Could you check a few things on this model? Use its own coordinates, in mm. Face numbers are marked on the shaded views. A direction names the side the tool comes from. Coordinates: 2 decimals unless noted, no trailing zeros. Write each loop counter-clockwise with the first axis right and the second up, starting at its lowest first coordinate (ties: lowest second). Pieces come first, ordered by that corner, then holes.
Item 1: For P1, Ø6, axis at y = 7.5, z = -1, coming from the +X side; P2, Ø3.5, axis at y = 10.5, z = 2.5, coming from the -X side; P3, Ø2.5, axis at x = 13, z = -1.5, coming from the +Y side, each with a flat end and sliding along its axis, tell me the tip position at first contact or that it passes through.
Item 2: Which directions (+Z, -Z, +X, -X, +Y, -Y) give clear straight access to the entire face, cutting with the end or side of a thin tool? Please do the marked faces 1, 2, 3 and 4.
Item 3: I want a section at C-C on z = 3.5. Please give me the cut outline in (x, y), then the cut area to 3 significant figures.
Item 4: I want a section at D-D on y = 20.5. Please give me the cut outline in (x, z).
Item 5: I want a section at B-B on x = 1. Please give me the cut outline in (y, z), then the cut area to 3 significant figures.
Item 6: If I drill on probe 1 along Y at (x, z) = (8, -1.25); probe 2 along X at (y, z) = (16.4, 0); probe 3 along X at (y, z) = (13.75, 0.5), over which ranges is the centre line in solid material (lowest first)?
Item 7: I want a section at A-A on x = -14. Please give me the cut outline in (y, z).
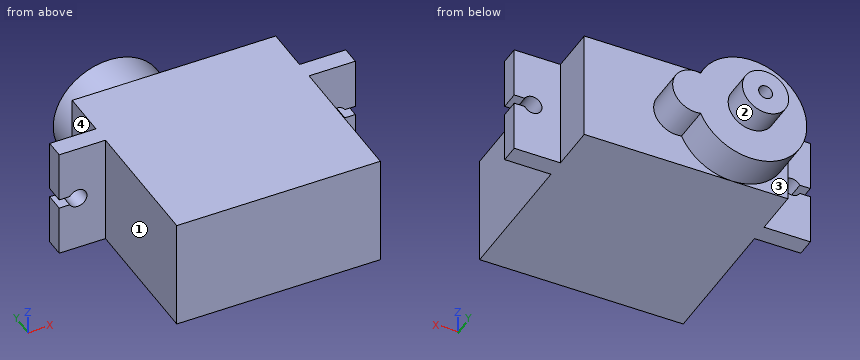
from build123d import *

# Parameters (mm, degrees)
SKETCH1_W           = 22
SKETCH1_H           = 12
BOSS_EXTRUDE1_DEPTH = 22
BOSS_EXTRUDE2_DEPTH = 4
SKETCH3_W           = 5
SKETCH3_H           = 2
BOSS_EXTRUDE3_DEPTH = 12
CUT_EXTRUDE1_REACH  = 26.104
SKETCH5_R           = 2.5
SKETCH5_R_2         = 0.75
BOSS_EXTRUDE4_DEPTH = 3


with BuildPart() as part:
    # Sketch1 → Boss-Extrude1 (new body)
    with BuildSketch(Plane(origin=(0, 0, 0), x_dir=(1, 0, 0), z_dir=(0, 1, 0))):
        Rectangle(SKETCH1_W, SKETCH1_H)
    extrude(amount=BOSS_EXTRUDE1_DEPTH)

    # Sketch2 → Boss-Extrude2 (add)
    with BuildSketch(Plane(origin=(0, 22, 0), x_dir=(1, 0, 0), z_dir=(0, 1, 0))):
        with BuildLine():
            ThreePointArc((0.479166667, 2.445144707), (-11, 0), (0.479166667, -2.445144707))
            ThreePointArc((0.479166667, -2.445144707), (3.5, 0), (0.479166667, 2.445144707))
        make_face()
    extrude(amount=BOSS_EXTRUDE2_DEPTH)

    # Sketch3 → Boss-Extrude3 (add)
    with BuildSketch(Plane.XY.offset(6)):
        with Locations((13.5, 16)):
            Rectangle(SKETCH3_W, SKETCH3_H)
    boss_extrude3 = extrude(amount=-BOSS_EXTRUDE3_DEPTH)

    # Sketch4 → Cut-Extrude1 (cut, up to next)
    with BuildSketch(Plane(origin=(0, 17, 0), x_dir=(1, 0, 0), z_dir=(0, 1, 0)), mode=Mode.PRIVATE) as cut_extrude1_sk1:
        with BuildLine():
            Line((14.866025404, 0.5), (16, 0.5))
            Line((16, 0.5), (16, -0.5))
            Line((16, -0.5), (14.866025404, -0.5))
            ThreePointArc((14.866025404, -0.5), (13, 0), (14.866025404, 0.5))
        make_face()
    cut_extrude1_tool1 = extrude(cut_extrude1_sk1.sketch, amount=-CUT_EXTRUDE1_REACH, mode=Mode.PRIVATE) & part.part
    cut_extrude1 = cut_extrude1_tool1.solids().sort_by_distance((14.368381, 17, 0))[0]
    add(cut_extrude1, mode=Mode.SUBTRACT)

    # Mirror1: Boss-Extrude3, Cut-Extrude1 across plane
    add(boss_extrude3.mirror(Plane(origin=(0, 0, 0), x_dir=(0, 0, 1), z_dir=(1, 0, 0))))
    add(cut_extrude1.mirror(Plane(origin=(0, 0, 0), x_dir=(0, 0, 1), z_dir=(1, 0, 0))), mode=Mode.SUBTRACT)

    # Sketch5 → Boss-Extrude4 (add)
    with BuildSketch(Plane(origin=(0, 26, 0), x_dir=(1, 0, 0), z_dir=(0, 1, 0))):
        with Locations(Location((-5, 0, 0), (0, 0, 270))):
            Circle(SKETCH5_R)
        with Locations(Location((-5, 0, 0), (0, 0, 270))):
            Circle(SKETCH5_R_2, mode=Mode.SUBTRACT)
    extrude(amount=BOSS_EXTRUDE4_DEPTH)


solid = part.part
Response values:
1. P1: stops at x = 11
1. P2: stops at x = -11
1. P3: stops at y = 17
2. face 1: +Z, -Z, -X, -Y
2. face 2: +Y
2. face 3: -Z, -X, +Y
2. face 4: +Z, -Z, -X, +Y
3. outline: (-16, 15) - (-11, 15) - (-11, 0) - (11, 0) - (11, 15) - (16, 15) - (16, 17) - (11, 17) - (11, 22) - (-0.13, 22) - (-0.13, 26) - (-9.87, 26) - (-9.87, 22) - (-11, 22) - (-11, 17) - (-16, 17) - close
3. area: 543 mm2
4. outline: (-11, -6) - (11, -6) - (11, 6) - (-11, 6) - close
5. outline: (0, -6) - (22, -6) - (22, -2.5) - (26, -2.5) - (26, 2.5) - (22, 2.5) - (22, 6) - (0, 6) - close
5. area: 284 mm2
6. probe 1: y = 0 to 22
6. probe 2: x = -13 to 13
6. probe 3: x = -11 to 11
7. outline: (15, -6) - (17, -6) - (17, -1) - (15, -1) - close; (15, 1) - (17, 1) - (17, 6) - (15, 6) - close
